Part model, mm, in its own coordinate system. A direction names the side the tool comes from. Give positions to 0.01 mm unless a question says otherwise; leave off trailing zeros. Write each loop counter-clockwise with the first axis right and the second up, starting at its lowest first coordinate (ties: lowest second). Pieces come first, ordered by that corner, then holes. Notation, with made-up numbers: M 61.25,-0.5 L 110.25,-0.5 A21 cw 110.25,26.5 Z; hole C 56.5,77 d3. An arc over 180 degrees is marked long. Write item = value, one per line. Start each with the question number.
from build123d import *

# Parameters (mm, degrees)
EXTRUDE_1_DEPTH      = 4
SKETCH_11_R          = 2
SKETCH_11_R_2        = 5
SKETCH_11_W          = 34
SKETCH_11_H          = 34
CUT_EXTRUDE_8_DEPTH  = 121.690720439
SKETCH_12_R          = 3.55
CUT_EXTRUDE_9_DEPTH  = 2
SKETCH_13_W          = 21.5
SKETCH_13_H          = 43.5
SKETCH_13_W_2        = 43.5
SKETCH_13_H_2        = 21.5
CUT_EXTRUDE_10_DEPTH = 2
SKETCH_14_R          = 1.5
CUT_EXTRUDE_11_DEPTH = 121.640996349


with BuildPart() as part:
    # 草圖1 → 填料-伸長1 (new body)
    with BuildSketch(Plane(origin=(0, 0, 0), x_dir=(1, 0, 0), z_dir=(0, 1, 0))):
        Polygon((-39.5, 49.5), (39.5, 49.5), (39.5, 27.5), (80.5, 27.5), (80.5, 49.5), (110, 49.5), (110, -49.5), (80.5, -49.5), (80.5, -27.5), (39.5, -27.5), (39.5, -49.5), (-39.5, -49.5), (-39.5, -27.5), (-80.5, -27.5), (-80.5, -49.5), (-110, -49.5), (-110, 49.5), (-80.5, 49.5), (-80.5, 27.5), (-39.5, 27.5), align=None)
    extrude(amount=EXTRUDE_1_DEPTH)

    # 草圖11 → 除料-伸長8 (cut, through all)
    with BuildSketch(Plane(origin=(0, 0, 0), x_dir=(1, 0, 0), z_dir=(0, 1, 0))):
        with Locations(Location((-106.5, 46, 0), (0, 0, 270))):
            Circle(SKETCH_11_R)
        with Locations(Location((-2.39e-07, 46, 0), (0, 0, 270))):
            Circle(SKETCH_11_R)
        with Locations(Location((106.5, 46, 0), (0, 0, 270))):
            Circle(SKETCH_11_R)
        with Locations(Location((-2.39e-07, -46, 0), (0, 0, 90))):
            Circle(SKETCH_11_R)
        with Locations(Location((-106.5, -46, 0), (0, 0, 90))):
            Circle(SKETCH_11_R)
        with Locations(Location((106.5, -46, 0), (0, 0, 90))):
            Circle(SKETCH_11_R)
        with Locations(Location((75, 0, 0), (0, 0, 270))):
            Circle(SKETCH_11_R_2)
        with Locations((3, 0)):
            Rectangle(SKETCH_11_W, SKETCH_11_H)
    extrude(amount=CUT_EXTRUDE_8_DEPTH, mode=Mode.SUBTRACT)

    # 草圖12 → 除料-伸長9 (cut)
    with BuildSketch(Plane(origin=(0, 4, 0), x_dir=(1, 0, 0), z_dir=(0, 1, 0))):
        with Locations((-106.5, 46)):
            Circle(SKETCH_12_R)
        with Locations((-2.39e-07, 46)):
            Circle(SKETCH_12_R)
        with Locations((-2.39e-07, -46)):
            Circle(SKETCH_12_R)
        with Locations((-106.5, -46)):
            Circle(SKETCH_12_R)
        with Locations((106.5, -46)):
            Circle(SKETCH_12_R)
        with Locations((106.5, 46)):
            Circle(SKETCH_12_R)
    extrude(amount=-CUT_EXTRUDE_9_DEPTH, mode=Mode.SUBTRACT)

    # 草圖13 → 除料-伸長10 (cut)
    with BuildSketch(Plane(origin=(0, 4, 0), x_dir=(1, 0, 0), z_dir=(0, 1, 0))):
        with Locations((-82.5, 0)):
            Rectangle(SKETCH_13_W, SKETCH_13_H)
        with Locations((0, -30.588054748)):
            Rectangle(SKETCH_13_W_2, SKETCH_13_H_2)
        with Locations((0, 30.588054748)):
            Rectangle(SKETCH_13_W_2, SKETCH_13_H_2)
    extrude(amount=-CUT_EXTRUDE_10_DEPTH, mode=Mode.SUBTRACT)

    # 草圖14 → 除料-伸長11 (cut, through all)
    with BuildSketch(Plane(origin=(0, 2, 0), x_dir=(1, 0, 0), z_dir=(0, 1, 0))):
        with Locations(Location((-74.5, 15.5, 0), (0, 0, 270))):
            Circle(SKETCH_14_R)
        with Locations(Location((-90.5, -15.5, 0), (0, 0, 270))):
            Circle(SKETCH_14_R)
        with Locations(Location((-15.5, -22.588054748, 0), (0, 0, 90))):
            Circle(SKETCH_14_R)
        with Locations(Location((15.5, -38.588054748, 0), (0, 0, 90))):
            Circle(SKETCH_14_R)
        with Locations(Location((15.5, 22.588054748, 0), (0, 0, 90))):
            Circle(SKETCH_14_R)
        with Locations(Location((-15.5, 38.588054748, 0), (0, 0, 90))):
            Circle(SKETCH_14_R)
    extrude(amount=-CUT_EXTRUDE_11_DEPTH, mode=Mode.SUBTRACT)


solid = part.part
Q1. Drop flat-ended pins along their axis: P1, Ø2, axis at x = -77.5, y = 3.5, coming from the -Z side; P2, Ø2, axis at x = -108, z = 44.5, coming from the +Y side. Give the stop position or say it passes through.
Q2. Slice it at D-D (x = 49.5). Give the cut face in (y, z).
Q3. Slice it at B-B (z = 0). Give the cut face in (x, y).
Q4. Probe line 1 along X through (y, z) = (0.4, 31); line 2 along X through (y, z) = (2.5, 10); line 3 along Z through (x, y) = (0, 2.9). List the from-to ranges inside material, lowest first.
Q5. Tool access for faces 1 (the face through (39.5, 2, 38)), 2 (the face through (95, 2, 49.5)), 3 (the face through (80.5, 2, -38)), 4 (the face through (3, 2, 17)), 5 (the face through (-108, 2, -48)): list every direction of +Z, -Z, +X, -X, +Y, -Y with a clear straight run to the whole face (end or side of a thin tool).
Q6. Two-plate mould, pull along Z, no slides. Class faces 6 (the face through (-80.5, 2, -39)), 7 (the face through (60, 2, 27.5)), 8 (the face through (104.517, 0.986, 46.26)): +Z half, -Z half, draft (parallel to the pull), parting line (faces both ways), or undercut.
Q7. Slice it at A-A (x = 75). Give the cut face in (y, z), and give its area (3 significant figures).
Q8. Slice it at C-C (y = 3.2). Give the number of separate pieces and of enclosed holes in the cut face, and give its area (3 significant figures).
Working result:
q1.P1 = -27.5
q1.P2 = 2
q2.outline = M 0,-27.5 L 4,-27.5 L 4,27.5 L 0,27.5 Z
q3.outline = M -110,0 L -14,0 L -14,4 L -71.75,4 L -71.75,2 L -93.25,2 L -93.25,4 L -110,4 Z; M 20,0 L 70,0 L 70,4 L 20,4 Z; M 80,0 L 110,0 L 110,4 L 80,4 Z
q4.line_1 = -110 to -80.5, -39.5 to 39.5, 80.5 to 110
q4.line_2 = -110 to -93.25, -71.75 to -14, 20 to 110
q4.line_3 = -42.45 to -41.34, -19.84 to -17, 17 to 19.84, 41.34 to 42.45
q5.face_1 = +Z, +Y, -Y
q5.face_2 = +Z, +X, -X, +Y, -Y
q5.face_3 = -Z, +Y, -Y
q5.face_4 = +Y, -Y
q5.face_5 = +Y
q6.face_6 = draft
q6.face_7 = +Z half
q6.face_8 = undercut
q7.outline = M 0,-27.5 L 4,-27.5 L 4,-5 L 0,-5 Z; M 0,5 L 4,5 L 4,27.5 L 0,27.5 Z
q7.area = 180 mm2
q8.separate_pieces = 5
q8.enclosed_holes = 5
q8.area = 13,900 mm2
